Source: CAD feature listing. Evaluate the final solid. Frame: model axes, mm. A direction names the side the tool comes from. Give positions to 0.01 mm unless a question says otherwise; leave off trailing zeros. Loops run counter-clockwise (first coordinate to the right, second up) from the corner with the lowest first, then second, coordinate; pieces in that order, holes last.
from build123d import *
from build123d.topology import SkipClean

# Parameters (mm, degrees)
CROQUIS1_W              = 60
CROQUIS1_H              = 50
CROQUIS1_R              = 1.5
SALIENTE_EXTRUIR1_DEPTH = 17.96
SALIENTE_EXTRUIR2_START = 4.7625
CROQUIS3_W              = 15
CROQUIS3_H              = 50
CROQUIS3_R              = 1.5
SALIENTE_EXTRUIR2_DEPTH = 4.7625
SALIENTE_EXTRUIR3_DEPTH = 4.7625
REDONDEO2_R             = 10
CORTAR_EXTRUIR1_DEPTH   = 5
CROQUIS6_W              = 10
CROQUIS6_H              = 50
CORTAR_EXTRUIR2_DEPTH   = 7


with BuildPart() as part:
    # Croquis1 → Saliente-Extruir1 (new body)
    with BuildSketch(Plane(origin=(0, 0, 0), x_dir=(0, 0, -1), z_dir=(1, 0, 0))):
        Rectangle(CROQUIS1_W, CROQUIS1_H)
        with Locations((-25, 20)):
            Circle(CROQUIS1_R, mode=Mode.SUBTRACT)
        with Locations(Location((25, 20, 0), (0, 0, 180))):
            Circle(CROQUIS1_R, mode=Mode.SUBTRACT)
        with Locations((25, -20)):
            Circle(CROQUIS1_R, mode=Mode.SUBTRACT)
        with Locations(Location((-25, -20, 0), (0, 0, 180))):
            Circle(CROQUIS1_R, mode=Mode.SUBTRACT)
    extrude(amount=SALIENTE_EXTRUIR1_DEPTH)

    # Croquis3 → Saliente-Extruir2 (add)
    # profile 1 of 2: a face of its own
    with SkipClean():  # the faces are left unmerged after this step: merging them gives an invalid solid
        with BuildSketch(Plane.ZY.offset(SALIENTE_EXTRUIR2_START)):
            with Locations((-22.5, 0)):
                Rectangle(CROQUIS3_W, CROQUIS3_H)
            with Locations((-25, -20)):
                Circle(CROQUIS3_R, mode=Mode.SUBTRACT)
            with Locations((-25, 20)):
                Circle(CROQUIS3_R, mode=Mode.SUBTRACT)
        # profile 2 of 2: a face of its own
        with BuildSketch(Plane.ZY.offset(SALIENTE_EXTRUIR2_START)):
            with Locations((22.5, 0)):
                Rectangle(CROQUIS3_W, CROQUIS3_H)
            with Locations((25, -20)):
                Circle(CROQUIS3_R, mode=Mode.SUBTRACT)
            with Locations((25, 20)):
                Circle(CROQUIS3_R, mode=Mode.SUBTRACT)
        extrude(amount=-SALIENTE_EXTRUIR2_DEPTH)

    # Croquis4 → Saliente-Extruir3 (add)
    with SkipClean():  # the faces are left unmerged after this step: merging them gives an invalid solid
        with BuildSketch(Plane.ZY):
            with BuildLine():
                Line((-5, 22.744997998), (-5, 25))
                Line((-5, 25), (5, 25))
                Line((5, 25), (5, 22.744997998))
                ThreePointArc((5, 22.744997998), (0, 8.5), (-5, 22.744997998))
            make_face()
            with BuildLine():
                Line((-5, -22.744997998), (-5, -25))
                Line((-5, -25), (5, -25))
                Line((5, -25), (5, -22.744997998))
                ThreePointArc((5, -22.744997998), (0, -8.5), (-5, -22.744997998))
            make_face()
        extrude(amount=SALIENTE_EXTRUIR3_DEPTH)

    # Redondeo2
    # the kernel refuses this fillet: 10 mm, written as the material it takes off along each edge
    with BuildSketch(Plane(origin=(17.96, -50, -30), x_dir=(-1, 0, 0), z_dir=(0, 1, 0)), Plane(origin=(17.96, 50, 30), x_dir=(-1, 0, 0), z_dir=(0, -1, 0))) as redondeo2_piece_1:
        with BuildLine():
            CenterArc((REDONDEO2_R, REDONDEO2_R), REDONDEO2_R, 180, 90)
            Line((0, REDONDEO2_R), (0, 0))
            Line((0, 0), (REDONDEO2_R, 0))
        make_face()
    extrude(amount=100, mode=Mode.SUBTRACT)
    with BuildSketch(Plane(origin=(17.96, 25, -55), x_dir=(0, -1, 0), z_dir=(0, 0, 1))) as redondeo2_piece_2:
        with BuildLine():
            CenterArc((REDONDEO2_R, -REDONDEO2_R), REDONDEO2_R, 90, 90)
            Line((0, -REDONDEO2_R), (0, 0))
            Line((0, 0), (REDONDEO2_R, 0))
        make_face()
    extrude(amount=110, mode=Mode.SUBTRACT)
    with BuildSketch(Plane(origin=(17.96, -25, 55), x_dir=(-1, 0, 0), z_dir=(0, 0, -1))) as redondeo2_piece_3:
        with BuildLine():
            CenterArc((REDONDEO2_R, REDONDEO2_R), REDONDEO2_R, 180, 90)
            Line((0, REDONDEO2_R), (0, 0))
            Line((0, 0), (REDONDEO2_R, 0))
        make_face()
    extrude(amount=110, mode=Mode.SUBTRACT)

    # Croquis5 → Cortar-Extruir1 (cut)
    with BuildSketch(Plane(origin=(17.96, 0, 0), x_dir=(0, 0, -1), z_dir=(1, 0, 0))):
        Polygon((-25, 23.464101615), (-28, 21.732050808), (-28, 18.267949192), (-25, 16.535898385), (-22, 18.267949192), (-22, 21.732050808), align=None)
        Polygon((25, 23.464101615), (22, 21.732050808), (22, 18.267949192), (25, 16.535898385), (28, 18.267949192), (28, 21.732050808), align=None)
        Polygon((25, -16.535898385), (22, -18.267949192), (22, -21.732050808), (25, -23.464101615), (28, -21.732050808), (28, -18.267949192), align=None)
        Polygon((-25, -16.535898385), (-28, -18.267949192), (-28, -21.732050808), (-25, -23.464101615), (-22, -21.732050808), (-22, -18.267949192), align=None)
    extrude(amount=-CORTAR_EXTRUIR1_DEPTH, mode=Mode.SUBTRACT)

    # Croquis6 → Cortar-Extruir2 (cut)
    with BuildSketch(Plane.ZY.offset(4.7625)):
        with Locations((25, 0)):
            Rectangle(CROQUIS6_W, CROQUIS6_H)
        with Locations((-25, 0)):
            Rectangle(CROQUIS6_W, CROQUIS6_H)
    extrude(amount=-CORTAR_EXTRUIR2_DEPTH, mode=Mode.SUBTRACT)


solid = part.part
1) Pull-direction query (Z, two-part tool) for faces 1 (the cylindrical face through (-2.348, -8.505, 0.276)), 2 (the flat face through (3, -25, 0)), 3 (the flat face through (-1, 0, 20)); classes: released by +Z, released by -Z, zero draft, split by the parting line, or undercut.
Checks:
face 1: undercut
face 2: zero draft
face 3: released by +Z
2) Reachability of faces 4 (the flat face through (12.96, 18.5, 25.7)), 5 (the flat face through (-2, 0, 15)), 6 (the flat face through (-2, 24, 5)) from +Z, -Z, +X, -X, +Y, -Y: full face, straight path, thin tool, end or side. Return the list, or none.
Checks:
face 4: +X
face 5: -X, +Y, -Y
face 6: -X, +Y
3) Cut plane B-B (z = 0). Return loops of the section in (x, y).
Checks:
outline: (-4.76, -25) - (7.96, -25) arc R10 ccw to (17.96, -15) - (17.96, 15) arc R10 ccw to (7.96, 25) - (-4.76, 25) - (-4.76, 8.5) - (0, 8.5) - (0, -8.5) - (-4.76, -8.5) - close
4) Contact query for flat-ended pins moving along their axis: P1, Ø6.5, axis at y = 20, z = -23.5, coming from the +X side; P2, Ø4, axis at x = 11, y = 15, coming from the -Z side; P3, Ø5.5, axis at x = -1, y = 4, coming from the +Z side; P4, Ø6, axis at x = -1, z = 14, coming from the -Y side. Output: stop coordinate, or through.
Checks:
P1: stops at x = 17.74
P2: stops at z = -29.95
P3: stops at z = 20
P4: stops at y = -25
5) Cut plane A-A (y = -2). Return loops of the section in (x, z), and give its area (3 significant figures).
Checks:
outline: (-4.76, -20) - (2.24, -20) - (2.24, -30) - (7.96, -30) arc R10 ccw to (17.96, -20) - (17.96, 20) arc R10 ccw to (7.96, 30) - (2.24, 30) - (2.24, 20) - (-4.76, 20) - (-4.76, 15) - (0, 15) - (0, -15) - (-4.76, -15) - close
area: 1,040 mm2
6) Cut plane C-C (y = 20). State how many separate pieces and enclosed holes the cut face has, and give its area (3 significant figures).
Checks:
separate pieces: 3
enclosed holes: 0
area: 942 mm2
7) Cut plane D-D (x = 0.75). Return loops of the section in (y, z).
Checks:
outline: (-25, -20) - (25, -20) - (25, 20) - (-25, 20) - close
8) Ray query, probe 1 along Y at (x, z) = (7.5, -25); probe 2 along Z at (x, y) = (5.5, 20.5); probe 3 along Z at (x, y) = (-2.25, -1). Return the intervals inside material, ascending.
Checks:
probe 1: y = -25 to -21.5, -18.5 to 18.5, 21.5 to 25
probe 2: z = -30 to -26.41, -23.59 to 23.59, 26.41 to 30
probe 3: z = -20 to -15, 15 to 20
